Here's how the part is built. I have some questions about the finished solid (model axes, mm). Face numbers are marked on the shaded views. A direction names the side the tool comes from. Coordinates: 2 decimals unless noted, no trailing zeros. Write each loop counter-clockwise with the first axis right and the second up, starting at its lowest first coordinate (ties: lowest second). Pieces come first, ordered by that corner, then holes.
Item 1: I'm going to push flat-ended pins straight in: pin 1 Ø5 at (x, y) = (140, 10) entering from -Z; pin 2 Ø4 at (x, y) = (125.5, 11.5) entering from +Z; pin 3 Ø4 at (x, z) = (158.5, 32.5) entering from +Y; pin 4 Ø5.5 at (x, z) = (3, 53.5) entering from -Y. Where does each tip first touch, or does it pass through?
Item 2: If we section it at B-B (z = 20): Please give me the cut outline in (x, y), then the cut area to 3 significant figures.
Item 3: For the marked faces 1 and 2, which set-ups out of +Z, -Z, +X, -X, +Y, -Y let a thin tool reach every point of the face, with its end or its side?
Item 4: If I drill on line 1 (X direction, y = 20, z = 71); line 2 (Y direction, x = 140, z = 2.95); line 3 (X direction, y = 10, z = 3), over which ranges is the centre line in solid material (lowest first)?
Item 5: If we section it at D-D (x = 109.5): Please give me the cut outline in (y, z), then the cut area to 3 significant figures.
Item 6: If we section it at C-C (x = 20): Please give me the cut outline in (y, z), then the cut area to 3 significant figures.
Item 7: We'd pull the mould along X, two halves only. Please class the marked faces 3, 4 and 5: +X half, -X half, draft (parallel to the pull), parting line (faces both ways), or undercut.
Item 8: If we section it at A-A (z = 65): Please give me the cut outline in (x, y).
Solid Edge part; units mm, degrees
sketch "Sketch1" plane through (0, 0, 0) normal (0, 0, 1) x (1, 0, 0)
  line L0 (160, 0) -> (160, 40)
  line L1 (160, 40) -> (0, 40)
  line L2 (0, 40) -> (0, 0)
  line L3 (0, 0) -> (160, 0)
extrude "Protrusion1" add sketch "Sketch1" along normal blind 5
sketch "Sketch2" plane through (75, 20, 5) normal (0, 0, 1) x (1, 0, 0)
  line L0 (80, 10) -> (85, 10)
  line L1 (85, 10) -> (85, -10)
  line L2 (85, -10) -> (80, -10)
  line L3 (80, -10) -> (80, 10)
  line L4 (-70, -10) -> (-70, 10)
  line L5 (-70, 10) -> (-75, 10)
  line L6 (-75, 10) -> (-75, -10)
  line L7 (-75, -10) -> (-70, -10)
extrude "ExtrudedProtrusion_2" add sketch "Sketch2" along normal blind 70
hole "Bohrung_1" [suppressed]
hole "Hole1" at (20, 10, 5) direction (0, 0, -1) diameter 4.2 end up to next start chamfer 1 start chamfer angle 45
hole "Hole2" at (140, 10, 5) direction (0, 0, -1) diameter 4.2 end up to next start chamfer 1 start chamfer angle 45
hole "Hole3" at (140, 30, 5) direction (0, 0, -1) diameter 4.2 end up to next start chamfer 1 start chamfer angle 45
hole "Bohrung_6" at (160, 20, 65) direction (-1, 0, 0) diameter 10 end through all
hole "Hole_7" at (157.5, 20, 75) direction (0, 0, -1) diameter 2.459 end up to next thread major 3 thread length 2
hole "Hole4" at (2.5, 20, 75) direction (0, 0, -1) diameter 2.459 end up to next thread major 3 thread length 2
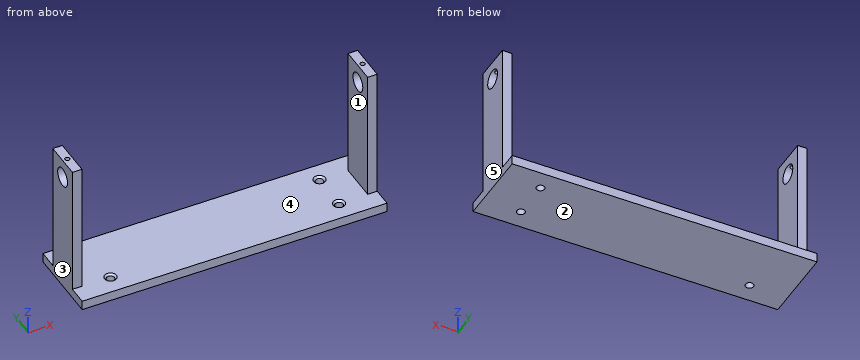
Answer list:
1. pin 1: stops at z = 0
1. pin 2: stops at z = 5
1. pin 3: stops at y = 30
1. pin 4: stops at y = 10
2. outline: (0, 10) - (5, 10) - (5, 30) - (0, 30) - close; (155, 10) - (160, 10) - (160, 30) - (155, 30) - close
2. area: 200 mm2
3. face 1: +Z, +Y, -Y
3. face 2: -Z, +X, -X, +Y, -Y
4. line 1: x = 0 to 1.27, 3.73 to 5, 155 to 156.27, 158.73 to 160
4. line 2: y = 0 to 7.9, 12.1 to 27.9, 32.1 to 40
4. line 3: x = 0 to 17.9, 22.1 to 137.9, 142.1 to 160
5. outline: (0, 0) - (40, 0) - (40, 5) - (0, 5) - close
5. area: 200 mm2
6. outline: (0, 0) - (7.9, 0) - (7.9, 4) - (6.9, 5) - (0, 5) - close; (12.1, 0) - (40, 0) - (40, 5) - (13.1, 5) - (12.1, 4) - close
6. area: 178 mm2
7. face 3: -X half
7. face 4: undercut
7. face 5: +X half
8. outline: (0, 10) - (5, 10) - (5, 15) - (0, 15) - close; (0, 25) - (5, 25) - (5, 30) - (0, 30) - close; (155, 10) - (160, 10) - (160, 15) - (155, 15) - close; (155, 25) - (160, 25) - (160, 30) - (155, 30) - close
